```python
from build123d import *

# Parameters (mm, degrees)
SKETCH1_W           = 200
SKETCH1_H           = 90
SKETCH1_R           = 14
SKETCH1_R_2         = 18.25
SKETCH1_R_3         = 2.25
SKETCH1_R_4         = 3.25
SKETCH1_R_5         = 2.5
BOSS_EXTRUDE1_DEPTH = 4
FILLET1_R           = 5
SKETCH3_R           = 35.6
SKETCH3_R_2         = 30
CUT_EXTRUDE1_DEPTH  = 3.5
SKETCH4_R           = 5
CUT_EXTRUDE2_DEPTH  = 5


with BuildPart() as part:
    # Sketch1 → Boss-Extrude1 (new body, symmetric)
    with BuildSketch(Plane.XY):
        Rectangle(SKETCH1_W, SKETCH1_H)
        with Locations((-55, 0)):
            Circle(SKETCH1_R, mode=Mode.SUBTRACT)
        with Locations((55, 0)):
            Circle(SKETCH1_R_2, mode=Mode.SUBTRACT)
        with Locations((65.142838282, -21.751386889)):
            Circle(SKETCH1_R_3, mode=Mode.SUBTRACT)
        with Locations((48.788342918, -23.182219831)):
            Circle(SKETCH1_R_3, mode=Mode.SUBTRACT)
        with Locations((35.340350937, -13.765834472)):
            Circle(SKETCH1_R_3, mode=Mode.SUBTRACT)
        with Locations((31.091327246, 2.091737826)):
            Circle(SKETCH1_R_3, mode=Mode.SUBTRACT)
        with Locations((38.029437252, 16.970562748)):
            Circle(SKETCH1_R_3, mode=Mode.SUBTRACT)
        with Locations((52.908262174, 23.908672754)):
            Circle(SKETCH1_R_3, mode=Mode.SUBTRACT)
        with Locations((68.765834472, 19.659649063)):
            Circle(SKETCH1_R_3, mode=Mode.SUBTRACT)
        with Locations((78.182219831, 6.211657082)):
            Circle(SKETCH1_R_3, mode=Mode.SUBTRACT)
        with Locations((76.751386889, -10.142838282)):
            Circle(SKETCH1_R_3, mode=Mode.SUBTRACT)
        with Locations((-90, 35)):
            Circle(SKETCH1_R_4, mode=Mode.SUBTRACT)
        with Locations((-20, 35)):
            Circle(SKETCH1_R_4, mode=Mode.SUBTRACT)
        with Locations((-90, -35)):
            Circle(SKETCH1_R_4, mode=Mode.SUBTRACT)
        with Locations((-20, -35)):
            Circle(SKETCH1_R_4, mode=Mode.SUBTRACT)
        with Locations((90, 35)):
            Circle(SKETCH1_R_4, mode=Mode.SUBTRACT)
        with Locations((90, -35)):
            Circle(SKETCH1_R_4, mode=Mode.SUBTRACT)
        with Locations((20, -35)):
            Circle(SKETCH1_R_4, mode=Mode.SUBTRACT)
        with Locations((20, 35)):
            Circle(SKETCH1_R_4, mode=Mode.SUBTRACT)
        with Locations((-75, 37)):
            Circle(SKETCH1_R_5, mode=Mode.SUBTRACT)
        with Locations((-92, 20)):
            Circle(SKETCH1_R_5, mode=Mode.SUBTRACT)
        with Locations((-92, -20)):
            Circle(SKETCH1_R_5, mode=Mode.SUBTRACT)
        with Locations((-75, -37)):
            Circle(SKETCH1_R_5, mode=Mode.SUBTRACT)
        with Locations((-35, -37)):
            Circle(SKETCH1_R_5, mode=Mode.SUBTRACT)
        with Locations((-18, -20)):
            Circle(SKETCH1_R_5, mode=Mode.SUBTRACT)
        with Locations((-18, 20)):
            Circle(SKETCH1_R_5, mode=Mode.SUBTRACT)
        with Locations((-35, 37)):
            Circle(SKETCH1_R_5, mode=Mode.SUBTRACT)
    extrude(amount=BOSS_EXTRUDE1_DEPTH, both=True)

    # Fillet1
    fillet1_edges = [part.edges().sort_by_distance(p)[0] for p in [
        (100, -45, 0),
        (-100, -45, 0),
        (-100, 45, 0),
        (100, 45, 0),
    ]]
    fillet(fillet1_edges, radius=FILLET1_R)

    # Sketch3 → Cut-Extrude1 (cut)
    with BuildSketch(Plane.XY.offset(4)):
        with Locations((-55, 0)):
            Circle(SKETCH3_R)
        with Locations((55, 0)):
            Circle(SKETCH3_R_2)
    extrude(amount=-CUT_EXTRUDE1_DEPTH, mode=Mode.SUBTRACT)

    # Sketch4 → Cut-Extrude2 (cut)
    with BuildSketch(Plane(origin=(0, 0, -4), x_dir=(-1, 0, 0), z_dir=(0, 0, -1))):
        with Locations((90, 35)):
            Circle(SKETCH4_R)
        with Locations((20, 35)):
            Circle(SKETCH4_R)
        with Locations((90, -35)):
            Circle(SKETCH4_R)
        with Locations((20, -35)):
            Circle(SKETCH4_R)
        with Locations((-90, -35)):
            Circle(SKETCH4_R)
        with Locations((-20, -35)):
            Circle(SKETCH4_R)
        with Locations((-20, 35)):
            Circle(SKETCH4_R)
        with Locations((-90, 35)):
            Circle(SKETCH4_R)
    extrude(amount=-CUT_EXTRUDE2_DEPTH, mode=Mode.SUBTRACT)


solid = part.part
```
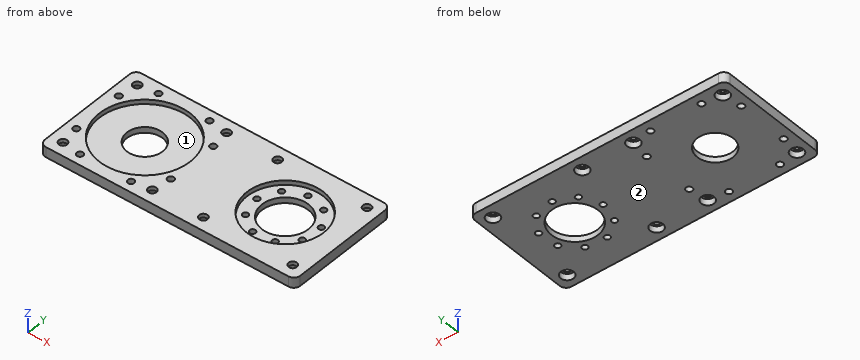
Model file for the job. Use its own axes, mm. Face numbers are marked on the shaded views. Coordinates: 2 decimals unless noted, no trailing zeros. Loops run counter-clockwise (first coordinate to the right, second up) from the corner with the lowest first, then second, coordinate; pieces in that order, holes last. Notation, with made-up numbers: (42, 67) - (95, 67) arc R17 ccw to (95, 82) - close; hole circle Ø6 at (29, -29). An arc over 180 degrees is marked (long way). Answer as a JSON object with one key per item and string values. Group by question number.
(1) Flat gauge pins, fed straight in: pin 1 (7 mm diameter, centred on x = 35.34, y = -13.77, fed in from +Z); pin 2 (3 mm diameter, centred on x = 91.5, y = -34.5, fed in from -Z); pin 3 (3 mm diameter, centred on x = -19.5, y = -37.5, fed in from -Z). Where does each tip first touch, or does it go through?
(2) Cut at A-A (x = 90). Give the cut face in (y, z).
(3) Probe line 1 along Y through (x, z) = (90, 1.7); line 2 along X through (y, z) = (-12, -0.5); line 3 along X through (y, z) = (-32.5, -3.5). List the from-to ranges inside material, lowest first.
(4) Cut at C-C (x = -81). Give the cut face in (y, z), then the cut area to 3 significant figures.
(5) Two-plate mould, pull along Y, no slides. Class the marked faces 1 and 2: released by +Y, released by -Y, zero draft, split by the parting line, or undercut.
(6) Cut at B-B (x = -48). Give the cut face in (y, z), then the cut area to 3 significant figures.
Geometry says:
{
 "1": {"pin 1": "stops at z = 0.5", "pin 2": "passes through", "pin 3": "stops at z = 1"},
 "2": {"outline": "(-45, -4) - (-40, -4) - (-40, 1) - (-38.25, 1) - (-38.25, 4) - (-45, 4) - close; (-31.75, 1) - (-30, 1) - (-30, -4) - (30, -4) - (30, 1) - (31.75, 1) - (31.75, 4) - (-31.75, 4) - close; (38.25, 1) - (40, 1) - (40, -4) - (45, -4) - (45, 4) - (38.25, 4) - close"},
 "3": {"line 1": "y = -45 to -38.25, -31.75 to 31.75, 38.25 to 45", "line 2": "x = -100 to -62.21, -47.79 to 33.95, 36.73 to 41.25, 68.75 to 75.48, 78.02 to 100", "line 3": "x = -100 to -94.33, -85.67 to -24.33, -15.67 to 15.67, 24.33 to 85.67, 94.33 to 100"},
 "4": {"outline": "(-45, -4) - (45, -4) - (45, 4) - (24.32, 4) - (24.32, 0.5) - (-24.32, 0.5) - (-24.32, 4) - (-45, 4) - close", "area": "550 mm^2"},
 "5": {"face 1": "undercut", "face 2": "zero draft"},
 "6": {"outline": "(-45, -4) - (-12.12, -4) - (-12.12, 0.5) - (-34.91, 0.5) - (-34.91, 4) - (-45, 4) - close; (12.12, -4) - (45, -4) - (45, 4) - (34.91, 4) - (34.91, 0.5) - (12.12, 0.5) - close", "area": "367 mm^2"}
}
